from build123d import *

# Parameters (mm, degrees)
RESSALTO_EXTRUS_O1_DEPTH = 33
FILETE1_START            = -1
FILETE1_DEPTH            = 35
FILETE1_2_DEPTH          = 33
CORTE_EXTRUS_O2_DEPTH    = 166.099690852
ESBO_O4_W                = 39.149175328
ESBO_O4_H                = 26.52668984
CORTE_EXTRUS_O3_DEPTH    = 166.099690852
ESBO_O5_W                = 74.27128815
ESBO_O5_H                = 142.377248688
CORTE_EXTRUS_O4_DEPTH    = 166.099690852
FILETE2_R                = 5
CORTE_EXTRUS_O5_DEPTH    = 163.400408603


with BuildPart() as part:
    # Esboço1 → Ressalto-extrusão1 (new body)
    with BuildSketch(Plane.XY):
        with BuildLine():
            Line((-14.089663978, 13.135393664), (-14.089663978, 28.135393664))
            Line((-14.089663978, 28.135393664), (-34.089663978, 28.135393664))
            Line((-34.089663978, 28.135393664), (-34.089663978, 158.135393664))
            Line((-34.089663978, 158.135393664), (25.910336022, 158.135393664))
            Line((25.910336022, 158.135393664), (25.910336022, 28.135393664))
            Line((25.910336022, 28.135393664), (5.910336022, 28.135393664))
            Line((5.910336022, 28.135393664), (5.910336022, 13.135393664))
            ThreePointArc((5.910336022, 13.135393664), (-4.089663978, 3.135393664), (-14.089663978, 13.135393664))
        make_face()
    extrude(amount=RESSALTO_EXTRUS_O1_DEPTH)

    # Filete1: read off the stored shape, not the designer's step
    # Filete1 outline → Filete1 (cut)
    with BuildSketch(Plane.XY.offset(FILETE1_START)):
        with BuildLine():
            Line((25.910336022, 28.135393664), (25.910336022, 38.135393664))
            ThreePointArc((25.910336022, 38.135393664), (22.981403834, 31.064325852), (15.910336022, 28.135393664))
            Line((15.910336022, 28.135393664), (25.910336022, 28.135393664))
        make_face()
        with BuildLine():
            Line((-34.089663978, 28.135393664), (-24.089663978, 28.135393664))
            ThreePointArc((-24.089663978, 28.135393664), (-31.160731789, 31.064325853), (-34.089663978, 38.135393664))
            Line((-34.089663978, 38.135393664), (-34.089663978, 28.135393664))
        make_face()
    extrude(amount=FILETE1_DEPTH, mode=Mode.SUBTRACT)

    # Filete1 2 outline → Filete1 2 (add)
    with BuildSketch(Plane.XY):
        with BuildLine():
            ThreePointArc((5.910336022, 18.135393664), (8.83926821, 25.206461475), (15.910336022, 28.135393664))
            Line((15.910336022, 28.135393664), (5.910336022, 28.135393664))
            Line((5.910336022, 28.135393664), (5.910336022, 18.135393664))
        make_face()
        with BuildLine():
            ThreePointArc((-24.089663978, 28.135393664), (-17.018596166, 25.206461476), (-14.089663978, 18.135393664))
            Line((-14.089663978, 18.135393664), (-14.089663978, 28.135393664))
            Line((-14.089663978, 28.135393664), (-24.089663978, 28.135393664))
        make_face()
    extrude(amount=FILETE1_2_DEPTH)

    # Esboço3 → Corte-extrusão2 (cut, through all)
    with BuildSketch(Plane.XY.offset(33)):
        with BuildLine():
            ThreePointArc((-34.089663978, 38.135393664), (-22.413633719, 98.135393664), (-34.089663978, 158.135393664))
            Line((-34.089663978, 158.135393664), (-34.089663978, 38.135393664))
        make_face()
        with BuildLine():
            ThreePointArc((25.910336022, 38.135393664), (14.234305764, 98.135393664), (25.910336022, 158.135393664))
            Line((25.910336022, 158.135393664), (25.910336022, 38.135393664))
        make_face()
    extrude(amount=-CORTE_EXTRUS_O2_DEPTH, mode=Mode.SUBTRACT)

    # Esboço4 → Corte-extrusão3 (cut, through all)
    with BuildSketch(Plane.XY.offset(33)):
        with Locations((-4.515076314, 14.872048744)):
            Rectangle(ESBO_O4_W, ESBO_O4_H)
    extrude(amount=-CORTE_EXTRUS_O3_DEPTH, mode=Mode.SUBTRACT)

    # Esboço5 → Corte-extrusão4 (cut, through all)
    with BuildSketch(Plane.XY.offset(33)):
        with Locations((19.722010356, 86.94676932)):
            Rectangle(ESBO_O5_W, ESBO_O5_H)
    extrude(amount=-CORTE_EXTRUS_O4_DEPTH, mode=Mode.SUBTRACT)

    # Filete2
    filete2_edges = [part.edges().sort_by_distance(p)[0] for p in [
        (-34.089663978, 158.135393664, 16.5),
    ]]
    fillet(filete2_edges, radius=FILETE2_R)

    # Esboço6 → Corte-extrusão5 (cut, through all)
    with BuildSketch(Plane(origin=(-17.413633719, 0, 0), x_dir=(0, 0, -1), z_dir=(1, 0, 0))):
        with BuildLine():
            Line((-19, 148.135393664), (-14, 148.135393664))
            ThreePointArc((-14, 148.135393664), (-11.171572875, 146.963820789), (-10, 144.135393664))
            Line((-10, 144.135393664), (-10, 122.135393664))
            ThreePointArc((-10, 122.135393664), (-11.171572875, 119.306966539), (-14, 118.135393664))
            Line((-14, 118.135393664), (-19, 118.135393664))
            ThreePointArc((-19, 118.135393664), (-21.828427125, 119.306966539), (-23, 122.135393664))
            Line((-23, 122.135393664), (-23, 144.135393664))
            ThreePointArc((-23, 144.135393664), (-21.828427125, 146.963820789), (-19, 148.135393664))
        make_face()
        with BuildLine():
            Line((-19, 108.135393664), (-14, 108.135393664))
            ThreePointArc((-14, 108.135393664), (-11.171572875, 106.963820789), (-10, 104.135393664))
            Line((-10, 104.135393664), (-10, 82.135393664))
            ThreePointArc((-10, 82.135393664), (-11.171572875, 79.306966539), (-14, 78.135393664))
            Line((-14, 78.135393664), (-19, 78.135393664))
            ThreePointArc((-19, 78.135393664), (-21.828427125, 79.306966539), (-23, 82.135393664))
            Line((-23, 82.135393664), (-23, 104.135393664))
            ThreePointArc((-23, 104.135393664), (-21.828427125, 106.963820789), (-19, 108.135393664))
        make_face()
        with BuildLine():
            Line((-19, 71.135393664), (-14, 71.135393664))
            ThreePointArc((-14, 71.135393664), (-11.171572875, 69.963820789), (-10, 67.135393664))
            Line((-10, 67.135393664), (-10, 45.135393664))
            ThreePointArc((-10, 45.135393664), (-11.171572875, 42.306966539), (-14, 41.135393664))
            Line((-14, 41.135393664), (-19, 41.135393664))
            ThreePointArc((-19, 41.135393664), (-21.828427125, 42.306966539), (-23, 45.135393664))
            Line((-23, 45.135393664), (-23, 67.135393664))
            ThreePointArc((-23, 67.135393664), (-21.828427125, 69.963820789), (-19, 71.135393664))
        make_face()
    extrude(amount=-CORTE_EXTRUS_O5_DEPTH, mode=Mode.SUBTRACT)


solid = part.part
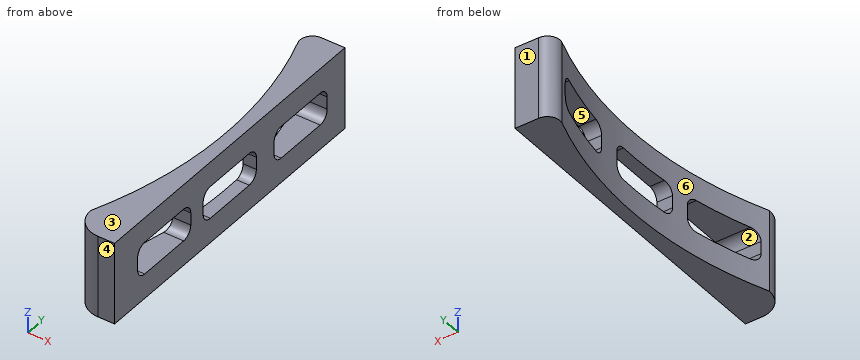
Verification items for the finished model (mm, model axes). Face numbers are marked on the shaded views. A direction names the side the tool comes from. Give positions to 0.01 mm unless a question says otherwise; leave off trailing zeros. Write each loop counter-clockwise with the first axis right and the second up, starting at its lowest first coordinate (ties: lowest second). Pieces come first, ordered by that corner, then holes.
(1) Access from +Z, -Z, +X, -X, +Y, -Y to the whole of each face (thin tool, end or side, straight path). Record for the marked faces 5 and 6.
(2) Material ranges on line 1 (Z direction, x = -25, y = 138.5); line 2 (Y direction, x = -19.25, z = 21); line 3 (X direction, y = 88, z = 4.5), recorded low to high.
(3) Cross-section at B-B (z = 21.5). Enter the section's corners in (x, y), plus the area to 3 significant figures.
(4) Mould release check, pull along Y, two halves, no side actions. Record for the marked faces 1, 2, 3 and 4: +Y half, -Y half, draft (parallel to the pull), parting line (faces both ways), or undercut.
(5) Gauge pin test, flat ends, axial feed: pin 1 (2.5 mm diameter, centred on x = -26, z = 16, fed in from -Y); pin 2 (8 mm diameter, centred on x = -31, y = 135, fed in from +Z); pin 3 (2 mm diameter, centred on y = 137, z = 23, fed in from -X); pin 4 (3 mm diameter, centred on y = 120.5, z = 4, fed in from -X). Record the tip position at first contact, or that the pin passes through.
(6) Cross-section at A-A (x = -21). Enter the section's corners in (y, z), plus the area to 3 significant figures.
(7) Cross-section at C-C (y = 141). Enter the section's corners in (x, z).
(8) Cross-section at D-D (z = 4). Enter the section's corners in (x, y).
Worked out:
1. face 5: +X, -X
1. face 6: +Z, -Z, -X
2. line 1: z = 0 to 10, 23 to 33
2. line 2: y = 28.14 to 41.67, 70.6 to 78.67, 107.6 to 118.67, 147.6 to 158.14
2. line 3: x = -22.73 to -17.41
3. outline: (-34.09, 38.14) arc R10 ccw to (-24.09, 28.14) - (-17.41, 28.14) - (-17.41, 42.01) - (-32.58, 42.01) arc R160 cw to start; (-31.56, 151.47) arc R160 cw to (-30.14, 147.26) - (-17.41, 147.26) - (-17.41, 158.14) - (-26.85, 158.14) arc R5 ccw to start; (-24.86, 70.26) - (-17.41, 70.26) - (-17.41, 79.01) - (-23.56, 79.01) arc R160 cw to start; (-23.78, 119.01) arc R160 cw to (-22.67, 107.26) - (-17.41, 107.26) - (-17.41, 119.01) - close
3. area: 481 mm2
4. face 1: +Y half
4. face 2: undercut
4. face 3: draft
4. face 4: -Y half
5. pin 1: stops at y = 28.16
5. pin 2: passes through
5. pin 3: stops at x = -27.46
5. pin 4: stops at x = -24.2
6. outline: (28.14, 0) - (158.14, 0) - (158.14, 33) - (28.14, 33) - close; hole (41.14, 14) arc R4 ccw to (45.14, 10) - (67.14, 10) arc R4 ccw to (71.14, 14) - (71.14, 19) arc R4 ccw to (67.14, 23) - (45.14, 23) arc R4 ccw to (41.14, 19) - close; hole (78.14, 14) arc R4 ccw to (82.14, 10) - (104.14, 10) arc R4 ccw to (108.14, 14) - (108.14, 19) arc R4 ccw to (104.14, 23) - (82.14, 23) arc R4 ccw to (78.14, 19) - close; hole (118.14, 14) arc R4 ccw to (122.14, 10) - (144.14, 10) arc R4 ccw to (148.14, 14) - (148.14, 19) arc R4 ccw to (144.14, 23) - (122.14, 23) arc R4 ccw to (118.14, 19) - close
6. area: 3,160 mm2
7. outline: (-28.26, 0) - (-17.41, 0) - (-17.41, 10) - (-28.26, 10) - close; (-28.26, 23) - (-17.41, 23) - (-17.41, 33) - (-28.26, 33) - close
8. outline: (-34.09, 38.14) arc R10 ccw to (-24.09, 28.14) - (-17.41, 28.14) - (-17.41, 158.14) - (-26.85, 158.14) arc R5 ccw to (-31.56, 151.47) arc R160 cw to start
